Answer from the drawing. Dimensions are ordinates in mm from the lowest x, y and z of the part. A direction names the side the tool comes from. Round coordinates to 2 decimals unless told otherwise and drop trailing zeros. Loops run counter-clockwise (first coordinate to the right, second up) from the corner with the lowest first, then second, coordinate; pieces in that order, holes last. Notation, with made-up numbers: (4, 59.25) - (41, 59.25) arc R18 cw to (41, 68.25) - close; hole circle Ø7 at (67.5, -34.75). An arc over 180 degrees is marked (long way). Answer as CSV lines item,"result".
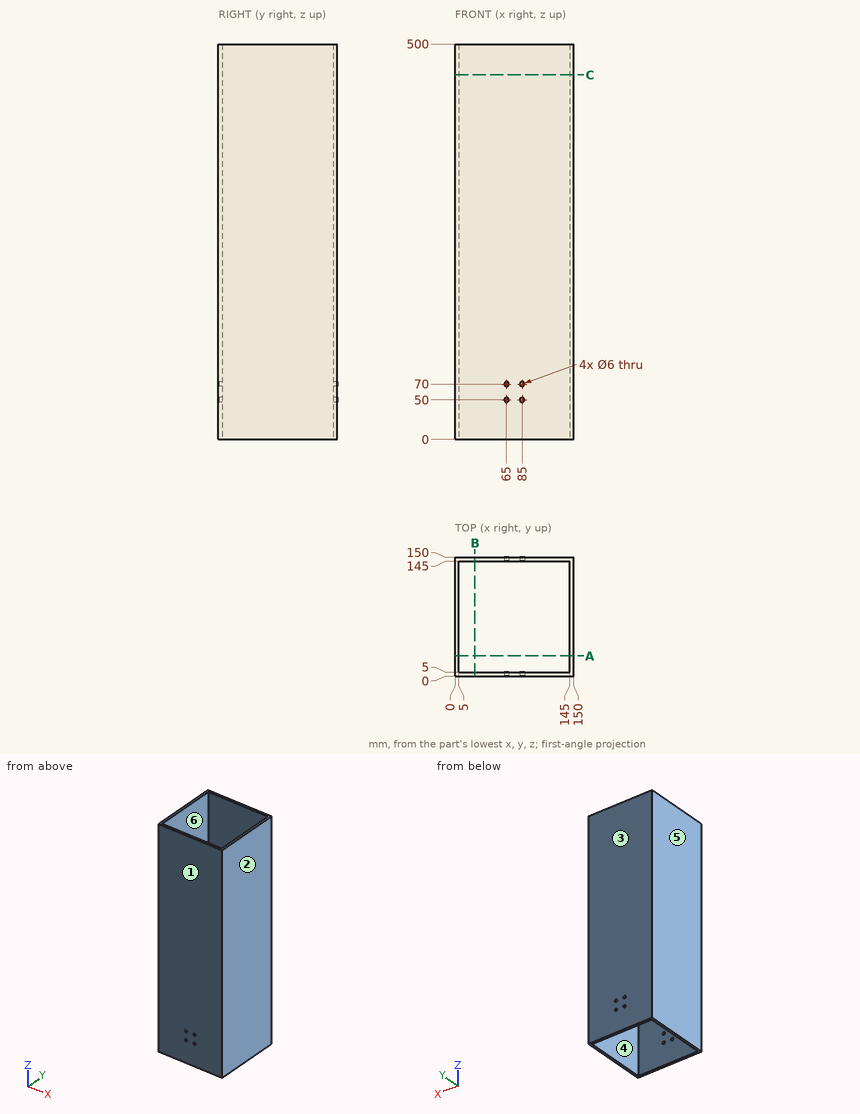
1) This flat-tipped pin is pushed along its axis until it touches: P1, Ø5, axis at x = 65, z = 70, coming from the -Y side. Where does it stop, or does it pass through?
Entries:
P1,"passes through"
2) Find the intervals of material crossed by line 1 (X direction, y = 147, z = 70); line 2 (Z direction, x = 85, y = 146.3); line 3 (X direction, y = 107.5, z = 300.5), in increasing order.
Entries:
line 1,"x = 0 to 62, 68 to 82, 88 to 150"
line 2,"z = 0 to 47, 53 to 67, 73 to 500"
line 3,"x = 0 to 5, 145 to 150"
3) The mould has two halves that part along Y. Classify the marked faces 1, 2, 3 and 4: pulls with the +Y half, pulls with the -Y half, needs draft (parallel to the pull), parting line crosses it, or undercut.
Entries:
face 1,"pulls with the -Y half"
face 2,"needs draft"
face 3,"pulls with the +Y half"
face 4,"undercut"
4) A tool of negligible diameter and unlimited length cuts with its end or side. For the marked faces 5 and 6, from which of +Z, -Z, +X, -X, +Y, -Y can it reach the whole face along a straight path? Write none if from no direction.
Entries:
face 5,"+Z, -Z, -X, +Y, -Y"
face 6,"+Z, -Z"
5) A cutting plane is placed at A-A, the plane y = 25.5. Determine the outline of the cut face in (x, z).
Entries:
outline,"(0, 0) - (5, 0) - (5, 500) - (0, 500) - close; (145, 0) - (150, 0) - (150, 500) - (145, 500) - close"
6) A cutting plane is placed at C-C, the plane z = 461. Determine the outline of the cut face in (x, y).
Entries:
outline,"(0, 0) - (150, 0) - (150, 150) - (0, 150) - close; hole (5, 5) - (145, 5) - (145, 145) - (5, 145) - close"
